from build123d import *

# Parameters (mm, degrees)
SKETCH1_R           = 7.5
BOSS_EXTRUDE1_DEPTH = 11
FILLET1_R           = 0.5
BOSS_EXTRUDE2_DEPTH = 9
SKETCH3_W           = 20
SKETCH3_H           = 20
CUT_EXTRUDE4_DEPTH  = 4
SKETCH5_R           = 1
BOSS_EXTRUDE3_DEPTH = 8
SKETCH5_3_R         = 0.7
CUT_EXTRUDE5_DEPTH  = 10
SKETCH5_4_R         = 0.8
CUT_EXTRUDE6_DEPTH  = 8.5
SKETCH6_R           = 2
SKETCH6_R_2         = 1.5
BOSS_EXTRUDE4_DEPTH = 0.7
CHAMFER1_SIZE       = 0.1
SKETCH9_W           = 11
SKETCH9_H           = 7
BOSS_EXTRUDE6_DEPTH = 3


with BuildPart() as part:
    # Sketch1 → Boss-Extrude1 (new body)
    with BuildSketch(Plane.XY):
        Circle(SKETCH1_R)
    extrude(amount=BOSS_EXTRUDE1_DEPTH)

    # Fillet1
    fillet1_edges = [part.edges().sort_by_distance(p)[0] for p in [
        (-7.5, 0, 0),
        (-7.5, 0, 11),
    ]]
    fillet(fillet1_edges, radius=FILLET1_R)

    # Sketch2 → Boss-Extrude2 (add)
    with BuildSketch(Plane.XY.offset(11)):
        with BuildLine():
            Line((-4, 6), (4, 6))
            ThreePointArc((4, 6), (4.707106781, 5.707106781), (5, 5))
            Line((5, 5), (5, -5))
            ThreePointArc((5, -5), (4.707106781, -5.707106781), (4, -6))
            Line((4, -6), (-4, -6))
            ThreePointArc((-4, -6), (-4.707106781, -5.707106781), (-5, -5))
            Line((-5, -5), (-5, 5))
            ThreePointArc((-5, 5), (-4.707106781, 5.707106781), (-4, 6))
        make_face()
    extrude(amount=BOSS_EXTRUDE2_DEPTH)

    # Sketch3 → Cut-Extrude4 (cut, symmetric)
    with BuildSketch(Plane.XY.offset(15.5)):
        Rectangle(SKETCH3_W, SKETCH3_H)
    extrude(amount=CUT_EXTRUDE4_DEPTH, both=True, mode=Mode.SUBTRACT)


with BuildPart() as cut_extrude4_piece_1:
    # of the separate pieces the step leaves, piece 1, a body of its own (cut_extrude4_pieces)
    add(part.part.solids().sort_by_distance((7.5, 0, 0.5))[0])



with BuildPart() as cut_extrude4_piece_2:
    # of the separate pieces the step leaves, piece 2, a body of its own (cut_extrude4_pieces)
    add(part.part.solids().sort_by_distance((5, -5, 19.5))[0])


with BuildPart() as cut_extrude4_piece_1_1:
    add(cut_extrude4_piece_1.part)

    add(cut_extrude4_piece_2.part)  # Boss-Extrude3 merges Cut-Extrude4 piece 2
    # Sketch5 → Boss-Extrude3 (add)
    with BuildSketch(Plane.XY.offset(11.5)):
        with Locations((-2.5, 3.8)):
            Circle(SKETCH5_R)
        with Locations((2.5, -3.8)):
            Circle(SKETCH5_R)
    extrude(amount=BOSS_EXTRUDE3_DEPTH)

    # Sketch5<3> → Cut-Extrude5 (cut)
    with BuildSketch(Plane.XY.offset(11.5)):
        with Locations((0, 4.5)):
            Circle(SKETCH5_3_R)
        with Locations((0, -4.5)):
            Circle(SKETCH5_3_R)
    extrude(amount=CUT_EXTRUDE5_DEPTH, mode=Mode.SUBTRACT)

    # Sketch5<4> → Cut-Extrude6 (cut)
    with BuildSketch(Plane.XY.offset(11.5)):
        with Locations((-2.5, 3.8)):
            Circle(SKETCH5_4_R)
        with Locations((2.5, -3.8)):
            Circle(SKETCH5_4_R)
    extrude(amount=CUT_EXTRUDE6_DEPTH, mode=Mode.SUBTRACT)

    # Sketch6 → Boss-Extrude4 (add)
    with BuildSketch(Plane.XY.offset(20)):
        Circle(SKETCH6_R)
        Circle(SKETCH6_R_2, mode=Mode.SUBTRACT)
    extrude(amount=BOSS_EXTRUDE4_DEPTH)

    # Chamfer1
    chamfer1_edges = [cut_extrude4_piece_1_1.edges().sort_by_distance(p)[0] for p in [
        (-3.3, 3.8, 20),
        (1.7, -3.8, 20),
    ]]
    chamfer(chamfer1_edges, length=CHAMFER1_SIZE)

    # Sketch9 → Boss-Extrude6 (add)
    with BuildSketch(Plane(origin=(0, 7.5, 0), x_dir=(1, 0, 0), z_dir=(0, 1, 0))):
        with Locations((0, -6)):
            Rectangle(SKETCH9_W, SKETCH9_H)
    extrude(amount=-BOSS_EXTRUDE6_DEPTH)


solid = cut_extrude4_piece_1_1.part
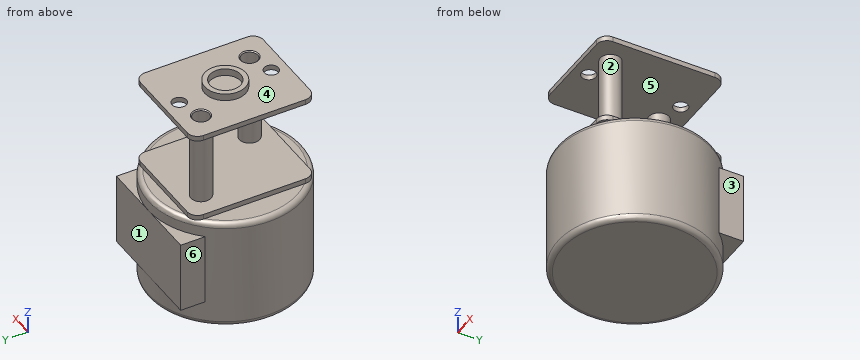
For this review, take the finished solid that the model builds, in its own axes (mm). Face numbers are marked on the shaded views. A direction names the side the tool comes from. Give positions to 0.01 mm unless a question says otherwise; leave off trailing zeros. Order: outer loops, then holes, each group sorted by start corner. A loop starts at its lowest first (then second) coordinate and runs counter-clockwise, first axis right, second up. Notation, with made-up numbers: (42.25, 34.25) - (70.25, 34.25) arc R25 ccw to (70.25, 66.25) - close; hole circle Ø6 at (11.5, 47). An arc over 180 degrees is marked (long way). Answer as a JSON object with one key per item and string values. Group by question number.
Item 1: Take a section at C-C on z = 5.25. Give the boundary of the cut face in (x, y), and give its area (3 significant figures).
Item 2: Take a section at A-A on z = 11.25. Give the boundary of the cut face in (x, y), and give its area (3 significant figures).
Item 3: Machinability: for the marked faces 1, 2 and 3, which of the approach directions +Z, -Z, +X, -X, +Y, -Y give a long, thin tool a straight path to every point of the face, cutting with its end or side? Answer none if there is none.
Item 4: Draft analysis for pull direction Z (two halves, no side actions). For the marked faces 4, 5 and 6, state which applies: pulls with the +Z half, pulls with the -Z half, needs draft (parallel to the pull), parting line crosses it, or undercut.
Item 5: Wall thickness on line 1 along Y through (x, z) = (0, 19.7); line 2 along Z through (x, y) = (4, 0.25); line 3 along Y through (x, z) = (2.5, 13.75): over which ranges is each line inside the solid? List them lowest first.
Item 6: Clearance check with flat-ended pins moving along their axes: pin 1 Ø8 at (x, y) = (5, -5.5) entering from +Z; pin 2 Ø1 at (y, z) = (-3, 2.5) entering from -X; pin 3 Ø3 at (y, z) = (4, 2.5) entering from +X. State where each tip first meets the part, or that it passes through.
Item 7: Take a section at B-B on z = 15.5. Give the boundary of the cut face in (x, y).
Reported:
{
 "1": {"outline": "(-5.5, 5.1) arc R7.5 ccw (long way) to (5.5, 5.1) - (5.5, 7.5) - (-5.5, 7.5) - close", "area": "185 mm^2"},
 "2": {"outline": "(-5, -5) arc R1 ccw to (-4, -6) - (4, -6) arc R1 ccw to (5, -5) - (5, 5) arc R1 ccw to (4, 6) - (-4, 6) arc R1 ccw to (-5, 5) - close", "area": "119 mm^2"},
 "3": {"face 1": "+Z, -Z, +X, -X, +Y", "face 2": "none", "face 3": "+Z, -Z, +X, +Y"},
 "4": {"face 4": "pulls with the +Z half", "face 5": "undercut", "face 6": "needs draft"},
 "5": {"line 1": "-6 to -5.2, -3.8 to 3.8, 5.2 to 6", "line 2": "0 to 11.5, 19.5 to 20", "line 3": "-4.8 to -4.6, -3 to -2.8"},
 "6": {"pin 1": "z = 20", "pin 2": "x = -7.07", "pin 3": "x = 7.07"},
 "7": {"outline": "circle Ø2 at (-2.5, 3.8); circle Ø2 at (2.5, -3.8); hole circle Ø1.6 at (-2.5, 3.8); hole circle Ø1.6 at (2.5, -3.8)"}
}
